Autodesk Inventor part; units mm, degrees
ref_plane "YZ Plane" through (0, 0, 0) normal (1, 0, 0) x (0, 1, 0)
ref_plane "XZ Plane" through (0, 0, 0) normal (0, 1, 0) x (-1, 0, 0)
ref_plane "XY Plane" through (0, 0, 0) normal (0, 0, 1) x (1, 0, 0)
sketch "スケッチ1" plane through (0, 0, 0) normal (0, 1, 0) x (-1, 0, 0)
  circle A0 centre (0, 0) radius 65
  circle A1 centre (0, 0) radius 60
  circle A2 centre (0, 0) radius 11
  circle A3 centre (0, 0) radius 16
  dimension "d0" = 130
  dimension "d1" = 120
  dimension "d3" = 32
  dimension "d18" = 22
extrude "押し出し1" add sketch "スケッチ1" against normal blind 5 contours A0 | A1 | A2 | A3
extrude "押し出し2" add sketch "スケッチ1" along normal blind 20 contours A3
extrude "押し出し3" add sketch "スケッチ1" along normal blind 25 contours A0
extrude "押し出し5" add sketch "スケッチ1" along normal blind 7 contours A2
sketch "スケッチ3" plane through (0, 7, 0) normal (0, 1, 0) x (1, 0, 0)
  circle A0 centre (0, 0) radius 2.5
  dimension "d15" = 5
extrude "押し出し6" cut sketch "スケッチ3" against normal blind 7
properties part number "tire out130 in 22 5mm inward"
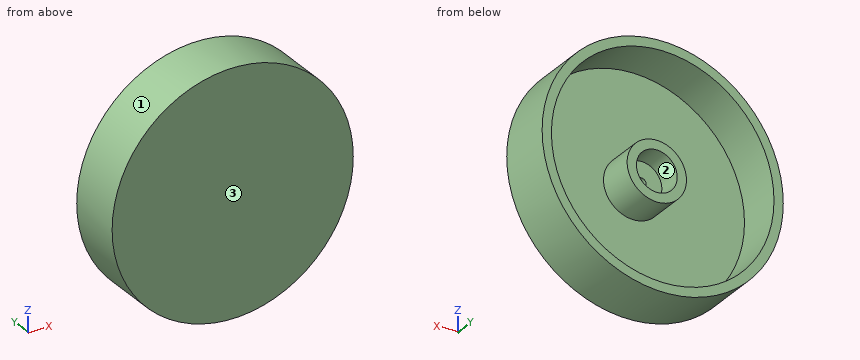
Can you work these out from the model? Positions are in its coordinate system, mm. Face numbers are marked on the shaded views. Give positions to 0.01 mm unless a question says otherwise; leave off trailing zeros. Write each loop counter-clockwise with the first axis right and the second up, starting at its lowest first coordinate (ties: lowest second). Pieces come first, ordered by that corner, then holes. Notation, with made-up numbers: (-16.75, 24.5) -> (13.25, 24.5) arc R20 ccw to (13.25, 63.5) -> close; hole circle Ø8 at (6.25, 19). An arc over 180 degrees is marked (long way). Answer as a JSON object with one key per item and string values. Group by question number.
Item 1: Please list where these lines run through material, in increasing order: line 1 (Z direction, x = 0, y = 3); line 2 (Z direction, x = 3.5, y = 8.5); line 3 (X direction, y = 18.5, z = -9). Write a range as [from, to].
Item 2: We'd pull the mould along X, two halves only. Please class the marked faces 1, 2 and 3: +X half, -X half, draft (parallel to the pull), parting line (faces both ways), or undercut.
Item 3: Suppose I cut it at C-C (z = 0). Please give me the cut outline in (x, y), plus the area to 3 significant figures.
Item 4: I'm going to push flat-ended pins straight in: P1, Ø4.5, axis at x = 0, z = 0, coming from the +Y side; P2, Ø6, axis at y = 6, z = -21.5, coming from the +X side; P3, Ø3, axis at x = 46, y = 0.5, coming from the +Z side. Where does each tip first touch, or does it pass through?
Item 5: Suppose I cut it at A-A (x = 0). Please give me the cut outline in (y, z).
Item 6: Suppose I cut it at D-D (y = 23). Please give me the cut outline in (x, z), plus the area to 3 significant figures.
Item 7: Suppose I cut it at B-B (y = 4.5). Please give me the cut outline in (x, z), plus the area to 3 significant figures.
Findings:
{
 "1": {"line 1": "z = [-65, -60], [-16, -2.5], [2.5, 16], [60, 65]", "line 2": "z = [-64.91, -59.9], [-15.61, -10.43], [10.43, 15.61], [59.9, 64.91]", "line 3": "x = [-64.37, -59.32], [-13.23, -6.32], [6.32, 13.23], [59.32, 64.37]"},
 "2": {"face 1": "parting line", "face 2": "undercut", "face 3": "draft"},
 "3": {"outline": "(-65, -5) -> (65, -5) -> (65, 25) -> (60, 25) -> (60, 0) -> (16, 0) -> (16, 20) -> (11, 20) -> (11, 7) -> (2.5, 7) -> (2.5, 0) -> (-2.5, 0) -> (-2.5, 7) -> (-11, 7) -> (-11, 20) -> (-16, 20) -> (-16, 0) -> (-60, 0) -> (-60, 25) -> (-65, 25) -> close", "area": "1,220 mm²"},
 "4": {"P1": "stops at y = 0", "P2": "stops at x = 62.31", "P3": "stops at z = 47.38"},
 "5": {"outline": "(-5, -65) -> (25, -65) -> (25, -60) -> (0, -60) -> (0, -16) -> (20, -16) -> (20, -11) -> (7, -11) -> (7, -2.5) -> (0, -2.5) -> (0, 2.5) -> (7, 2.5) -> (7, 11) -> (20, 11) -> (20, 16) -> (0, 16) -> (0, 60) -> (25, 60) -> (25, 65) -> (-5, 65) -> close"},
 "6": {"outline": "circle Ø130 at (0, 0); hole circle Ø120 at (0, 0)", "area": "1,960 mm²"},
 "7": {"outline": "circle Ø130 at (0, 0); circle Ø32 at (0, 0); hole circle Ø120 at (0, 0); hole circle Ø5 at (0, 0)", "area": "2,750 mm²"}
}
